Read the model definition and answer for the solid it produces. Units are mm, in the model's axes. Face numbers are marked on the shaded views. A direction names the side the tool comes from. Give positions to 0.01 mm unless a question says otherwise; leave off trailing zeros. Loops run counter-clockwise (first coordinate to the right, second up) from the corner with the lowest first, then second, coordinate; pieces in that order, holes last. Notation, with made-up numbers: (-2.5, -6) - (12.5, -6) arc R27 ccw to (12.5, 19) - close; hole circle Ø10 at (20, 86.25). An arc over 180 degrees is marked (long way). Use a Markdown table: item, result. Add a question column.
Item 1: Each of these flat-tipped pins is pushed along its axis until it touches: P1, Ø1.5, axis at y = -1, z = -1, coming from the -X side; P2, Ø1.5, axis at x = -9.5, y = -2, coming from the -Z side; P3, Ø1.5, axis at x = 7.5, y = -0.5, coming from the +Z side. Where does it stop, or does it pass through?
Item 2: A cutting plane is placed at A-A (y = -2.1). Determine the outline of the cut face in (x, z).
Item 3: A cutting plane is placed at D-D (z = -0.25). Determine the outline of the cut face in (x, y), plus the area to 3 significant figures.
Item 4: For a pull along X with two mould halves and no side action, classify the marked faces 1, 2, 3 and 4 as +X half, -X half, draft (parallel to the pull), parting line (faces both ways), or undercut.
Item 5: A cutting plane is placed at C-C (z = 3.5). Determine the outline of the cut face in (x, y).
Item 6: Which of the six approach directions +Z, -Z, +X, -X, +Y, -Y give full straight-line access (tool end or side, diameter ignored) to the marked faces 5, 6 and 7?
Item 7: Consider probe 1 along X at (y, z) = (-2.4, -1); probe 2 along Z at (x, y) = (0, -0.85); probe 3 along Z at (x, y) = (-1, -1.45). Determine where each line is inside the solid, lowest interval first. Write a range as [from, to].
Item 8: A cutting plane is placed at B-B (x = 0). Determine the outline of the cut face in (y, z), plus the area to 3 significant figures.
from build123d import *

# Parameters (mm, degrees)
F0_R     = 2.5
F1_DEPTH = 3


# Not quite as in the source:
# - a feature names something its author has since deleted; it is built from what else it names


with BuildPart() as f1:
    # F0 (on Front) → F1 (new body)
    with BuildSketch(Plane.XZ):
        with BuildLine():
            Line((7.5, 0), (11, 0))
            ThreePointArc((11, 0), (0, 11), (-11, 0))
            Line((-11, 0), (-7.5, 0))
            Line((-7.5, 0), (-7.5, -3))
            Line((-7.5, -3), (-4.5, -3))
            Line((-4.5, -3), (-4.5, 0))
            Line((-4.5, 0), (-1.5, 0))
            Line((-1.5, 0), (-1.5, -3))
            Line((-1.5, -3), (1.5, -3))
            Line((1.5, -3), (1.5, 0))
            Line((1.5, 0), (4.5, 0))
            Line((4.5, 0), (4.5, -3))
            Line((4.5, -3), (7.5, -3))
            Line((7.5, -3), (7.5, 0))
        make_face()
        with Locations((0, 5)):
            Circle(F0_R, mode=Mode.SUBTRACT)
    extrude(amount=F1_DEPTH)


solid = f1.part
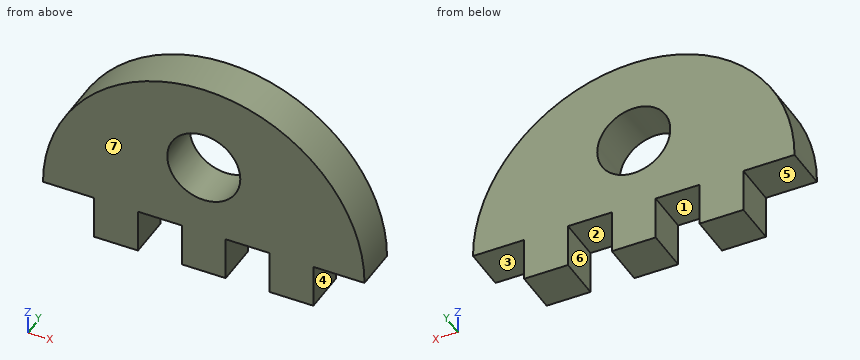
Geometry says:
| question | item | result |
|---|---|---|
| 1 | P1 | x = -7.5 |
| 1 | P2 | z = 0 |
| 1 | P3 | z = 8.69 |
| 2 | outline | (-11, 0) - (-7.5, 0) - (-7.5, -3) - (-4.5, -3) - (-4.5, 0) - (-1.5, 0) - (-1.5, -3) - (1.5, -3) - (1.5, 0) - (4.5, 0) - (4.5, -3) - (7.5, -3) - (7.5, 0) - (11, 0) arc R11 ccw to start; hole circle Ø5 at (0, 5) |
| 3 | outline | (-7.5, -3) - (-4.5, -3) - (-4.5, 0) - (-7.5, 0) - close; (-1.5, -3) - (1.5, -3) - (1.5, 0) - (-1.5, 0) - close; (4.5, -3) - (7.5, -3) - (7.5, 0) - (4.5, 0) - close |
| 3 | area | 27.0 mm² |
| 4 | face 1 | undercut |
| 4 | face 2 | undercut |
| 4 | face 3 | draft |
| 4 | face 4 | +X half |
| 5 | outline | (-10.43, -3) - (-2, -3) - (-2, 0) - (-10.43, 0) - close; (2, -3) - (10.43, -3) - (10.43, 0) - (2, 0) - close |
| 6 | face 5 | -Z, -X, +Y, -Y |
| 6 | face 6 | -Z, +Y, -Y |
| 6 | face 7 | +Z, -Z, +X, -X, -Y |
| 7 | probe 1 | [-7.5, -4.5], [-1.5, 1.5], [4.5, 7.5] |
| 7 | probe 2 | [-3, 2.5], [7.5, 11] |
| 7 | probe 3 | [-3, 2.71], [7.29, 10.95] |
| 8 | outline | (-3, -3) - (0, -3) - (0, 2.5) - (-3, 2.5) - close; (-3, 7.5) - (0, 7.5) - (0, 11) - (-3, 11) - close |
| 8 | area | 27.0 mm² |
